from build123d import *

# Parameters (mm, degrees)
SKETCH_1_R          = 2
EXTRUDE_1_DEPTH     = 6
CUT_EXTRUDE_START   = -4
CUT_EXTRUDE_2_DEPTH = 2
CUT_EXTRUDE_START_2 = 6
CUT_EXTRUDE_3_DEPTH = 2


with BuildPart() as part:
    # 草图1 → 凸台-拉伸1 (new, symmetric)
    with BuildSketch(Plane.XY):
        with BuildLine():
            Line((-30.5, 4.974937186), (-0.8, 7.959899497))
            ThreePointArc((-0.8, 7.959899497), (8, 0), (-0.8, -7.959899497))
            Line((-0.8, -7.959899497), (-30.5, -4.974937186))
            ThreePointArc((-30.5, -4.974937186), (-35, 0), (-30.5, 4.974937186))
        make_face()
        with Locations((-30, 0)):
            Circle(SKETCH_1_R, mode=Mode.SUBTRACT)
        with BuildLine():
            Line((-23.2, 1.989974874), (-13.3, 2.984962311))
            ThreePointArc((-13.3, 2.984962311), (-10, 0), (-13.3, -2.984962311))
            Line((-13.3, -2.984962311), (-23.2, -1.989974874))
            ThreePointArc((-23.2, -1.989974874), (-25, 0), (-23.2, 1.989974874))
        make_face(mode=Mode.SUBTRACT)
        with BuildLine():
            Line((2.5, 3.122498999), (2.5, -3.122498999))
            ThreePointArc((2.5, -3.122498999), (-4, 0), (2.5, 3.122498999))
        make_face(mode=Mode.SUBTRACT)
    extrude(amount=EXTRUDE_1_DEPTH, both=True)

    # 草图2 → 切除-拉伸2 (cut)
    with BuildSketch(Plane.XY.offset(CUT_EXTRUDE_START)):
        with BuildLine():
            Line((-30.5, -4.974937186), (-0.8, -7.959899497))
            ThreePointArc((-0.8, -7.959899497), (-8, 0), (-0.8, 7.959899497))
            Line((-0.8, 7.959899497), (-30.5, 4.974937186))
            ThreePointArc((-30.5, 4.974937186), (-35, 0), (-30.5, -4.974937186))
        make_face()
    extrude(amount=-CUT_EXTRUDE_2_DEPTH, mode=Mode.SUBTRACT)

    # 草图2<2> → 切除-拉伸3 (cut)
    with BuildSketch(Plane.XY.offset(CUT_EXTRUDE_START_2)):
        with BuildLine():
            Line((-30.5, -4.974937186), (-0.8, -7.959899497))
            ThreePointArc((-0.8, -7.959899497), (-8, 0), (-0.8, 7.959899497))
            Line((-0.8, 7.959899497), (-30.5, 4.974937186))
            ThreePointArc((-30.5, 4.974937186), (-35, 0), (-30.5, -4.974937186))
        make_face()
    extrude(amount=-CUT_EXTRUDE_3_DEPTH, mode=Mode.SUBTRACT)


solid = part.part
Design review of the part built by this model. Coordinates are the model's own, in mm. A direction names the side the tool comes from. Round coordinates to 2 decimals unless told otherwise and drop trailing zeros. Write each loop counter-clockwise with the first axis right and the second up, starting at its lowest first coordinate (ties: lowest second). Pieces come first, ordered by that corner, then holes. Notation, with made-up numbers: M 32,30.25 L 79,30.25 A32 cw 79,67.25 Z; hole C 34.25,-12 d8. An arc over 180 degrees is marked long. One line per item, written item: value. Start each with the question number.
1. Clearance check with flat-ended pins moving along their axes: P1, Ø1.9, axis at y = 1.5, z = 0.5, coming from the -X side; P2, Ø1.5, axis at x = -15.5, z = -2.5, coming from the +Y side; P3, Ø6.5, axis at x = -30, y = 0, coming from the -Z side; P4, Ø5.5, axis at x = -13, y = 0, coming from the +Z side. State where each tip first meets the part, or that it passes through.
2. Take a section at A-A on y = 0. State the section outline as (x, z) points.
3. To check wall thickness, follow probe 1 along X at (y, z) = (0, 3.25); probe 2 along Y at (x, z) = (0, 1.75); probe 3 along X at (y, z) = (1.75, 0.75). State the ranges of each line that lie inside material, in increasing order. Write a range as from..to.
4. Take a section at B-B on z = -3.25. State the section outline as (x, y) points.
5. Take a section at D-D on y = 2.5. State the section outline as (x, z) points.
6. Take a section at C-C on x = -3. State the section outline as (y, z) points, then the cut area to 3 significant figures.
7. Draft analysis for pull direction Y (two halves, no side actions). For faces 1 (the face through (-18, -3, 4)), 2 (the face through (-15.44, -6.49, 0.06)), 3 (the face through (-4, 0, 0)), 4 (the face through (-35, 0, 0)), state which applies: pulls with the +Y half, pulls with the -Y half, needs draft (parallel to the pull), parting line crosses it, or undercut.
8. For faces 5 (the face through (4, 0, 6)), 6 (the face through (-18.32, 2.48, 0.06)), list the 3-axis set-ups (+Z, -Z, +X, -X, +Y, -Y) from which the entire face can be reached by the end or side of a thin tool; tool diameter is ignored.
Computed:
1. P1: stops at x = -34.97
1. P2: stops at y = 6.56
1. P3: stops at z = -4
1. P4: passes through
2. outline: M -35,-4 L -32,-4 L -32,4 L -35,4 Z; M -28,-4 L -25,-4 L -25,4 L -28,4 Z; M -10,-4 L -8,-4 L -8,-6 L -4,-6 L -4,6 L -8,6 L -8,4 L -10,4 Z; M 2.5,-6 L 8,-6 L 8,6 L 2.5,6 Z
3. probe 1: x = -35..-32, -28..-25, -10..-4, 2.5..8
3. probe 2: y = -8..-4, 4..8
3. probe 3: x = -34.68..-30.97, -29.03..-23.97, -10.56..-3.6, 2.5..7.81
4. outline: M -30.5,-4.97 L -0.8,-7.96 A8 ccw long -0.8,7.96 L -30.5,4.97 A5 ccw Z; hole C -30,0 d4; hole M -23.2,-1.99 L -13.3,-2.98 A3 ccw long -13.3,2.98 L -23.2,1.99 A2 ccw Z; hole M 2.5,-3.12 L 2.5,3.12 A4 ccw long Z
5. outline: M -34.33,-4 L -18.13,-4 L -18.13,4 L -34.33,4 Z; M -11.34,-4 L -7.6,-4 L -7.6,-6 L -3.12,-6 L -3.12,6 L -7.6,6 L -7.6,4 L -11.34,4 Z; M 2.5,-6 L 7.6,-6 L 7.6,6 L 2.5,6 Z
6. outline: M -7.74,-4 L -7.42,-4 L -7.42,-6 L -2.65,-6 L -2.65,6 L -7.42,6 L -7.42,4 L -7.74,4 Z; M 2.65,-6 L 7.42,-6 L 7.42,-4 L 7.74,-4 L 7.74,4 L 7.42,4 L 7.42,6 L 2.65,6 Z
6. area: 120 mm²
7. face 1: needs draft
7. face 2: pulls with the -Y half
7. face 3: undercut
7. face 4: parting line crosses it
8. face 5: +Z, +X, -X, +Y, -Y
8. face 6: +Z, -Z
